Check sheet for the drawn part. Datum: minimum x, y, z corner. Units: mm. Give positions to 0.01 mm unless a question says otherwise; leave off trailing zeros. Loops run counter-clockwise (first coordinate to the right, second up) from the corner with the lowest first, then second, coordinate; pieces in that order, holes last. Notation, with made-up numbers: (64, 56) - (109, 56) arc R34 ccw to (109, 91) - close; hole circle Ø7 at (81.5, 32). An arc over 180 degrees is marked (long way). Answer in a Markdown table with one row per item.
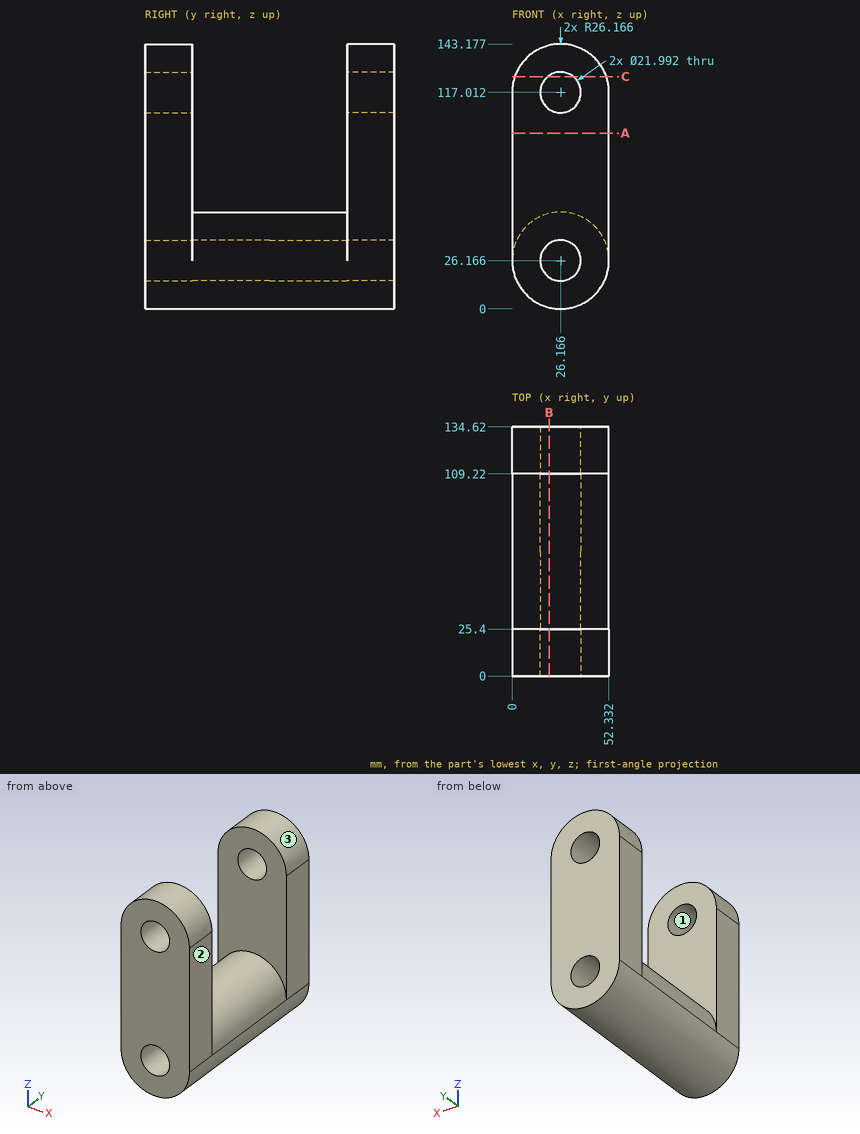
Q1. Sectioned sample at C-C (z = 125.5). Record the cut outline in (x, y) (1 decimal).
Completed:
| item | result |
|---|---|
| outline | (1.4, 0) - (19.2, 0) - (19.2, 25.4) - (1.4, 25.4) - close; (1.4, 109.2) - (19.2, 109.2) - (19.2, 134.6) - (1.4, 134.6) - close; (33.2, 0) - (50.9, 0) - (50.9, 25.4) - (33.2, 25.4) - close; (33.2, 109.2) - (50.9, 109.2) - (50.9, 134.6) - (33.2, 134.6) - close |
Q2. Go/stop test with flat-tipped pins: P1, Ø6, axis at x = 13, y = 98.5, coming from the -Z side (1 decimal); P2, Ø2, axis at x = 20, y = 50.5, coming from the +Z side; P3, Ø17.5, axis at x = 26.17, z = 117.01, coming from the +Y side; P4, Ø5, axis at x = 16.5, y = 98.5, coming from the -Z side. Record where each tip stops, or that it passes through.
Completed:
| item | result |
|---|---|
| P1 | z = 2.1 |
| P2 | z = 51.82 |
| P3 | through |
| P4 | z = 1 |
Q3. Thickness scan on line 1 (Z direction, x = 25.5, y = 123) (1 decimal); line 2 (Y direction, x = 2, z = 118.5); line 3 (Z direction, x = 34, y = 63). Record the ranges inside material, lowest first.
Completed:
| item | result |
|---|---|
| line 1 | 0 to 15.2, 37.1 to 106, 128 to 143.2 |
| line 2 | 0 to 25.4, 109.22 to 134.62 |
| line 3 | 1.2 to 18.45, 33.88 to 51.13 |
Q4. Sectioned sample at B-B (x = 20). Record the cut outline in (y, z) (1 decimal).
Completed:
| item | result |
|---|---|
| outline | (0, 0.7) - (134.6, 0.7) - (134.6, 17.1) - (0, 17.1) - close; (0, 35.3) - (134.6, 35.3) - (134.6, 107.9) - (109.2, 107.9) - (109.2, 51.6) - (25.4, 51.6) - (25.4, 107.9) - (0, 107.9) - close; (0, 126.1) - (25.4, 126.1) - (25.4, 142.4) - (0, 142.4) - close; (109.2, 126.1) - (134.6, 126.1) - (134.6, 142.4) - (109.2, 142.4) - close |
Q5. Sectioned sample at A-A (z = 95). Record the cut outline in (x, y).
Completed:
| item | result |
|---|---|
| outline | (0, 0) - (52.33, 0) - (52.33, 25.4) - (0, 25.4) - close; (0, 109.22) - (52.33, 109.22) - (52.33, 134.62) - (0, 134.62) - close |
Q6. Draft check along Z on the marked faces 1, 2 and 3. Enter one of: +Z half, -Z half, draft (parallel to the pull), parting line (faces both ways), or undercut.
Completed:
| item | result |
|---|---|
| face 1 | undercut |
| face 2 | draft |
| face 3 | +Z half |
